```python
from build123d import *

# Parameters (mm, degrees)
SKETCH1_R                = 3
BOSS_EXTRUDE1_DEPTH      = 17
CUT_EXTRUDE3_DEPTH       = 10.2
BOSS_EXTRUDE2_DEPTH      = 2
SKETCH4_R                = 1.5
BOSS_EXTRUDE3_DEPTH      = 18.5
BOSS_EXTRUDE4_DEPTH      = 2
BOSS_EXTRUDE4_DEPTH_BACK = 1
SKETCH6_R                = 2
SKETCH6_R_2              = 1
SKETCH7_R                = 1.1
CUT_EXTRUDE4_DEPTH       = 3


with BuildPart() as part:
    # Sketch1 → Boss-Extrude1 (new body)
    with BuildSketch(Plane(origin=(0, 0, 0), x_dir=(1, 0, 0), z_dir=(0, 1, 0))):
        with Locations(Location((0, 0, 0), (0, 0, 270))):
            Circle(SKETCH1_R)
    extrude(amount=BOSS_EXTRUDE1_DEPTH)

    # Sketch2 → Cut-Extrude3 (cut)
    with BuildSketch(Plane(origin=(0, 17, 0), x_dir=(1, 0, 0), z_dir=(0, 1, 0))):
        with BuildLine():
            Line((1.2, 1.204159458), (1.2, -1.204159458))
            ThreePointArc((1.2, -1.204159458), (-1.7, 0), (1.2, 1.204159458))
        make_face()
    extrude(amount=-CUT_EXTRUDE3_DEPTH, mode=Mode.SUBTRACT)

    # Sketch3 → Boss-Extrude2 (add)
    with BuildSketch(Plane(origin=(0, 0, 0), x_dir=(-1, 0, 0), z_dir=(0, -1, 0))):
        Polygon((5.196152423, 0), (2.598076211, 4.5), (-2.598076211, 4.5), (-5.196152423, 0), (-2.598076211, -4.5), (2.598076211, -4.5), align=None)
    extrude(amount=-BOSS_EXTRUDE2_DEPTH)

    # Sketch4 → Boss-Extrude3 (add)
    with BuildSketch(Plane(origin=(0, 0, 0), x_dir=(-1, 0, 0), z_dir=(0, -1, 0))):
        with Locations(Location((0, 0, 0), (0, 0, 90))):
            Circle(SKETCH4_R)
    extrude(amount=BOSS_EXTRUDE3_DEPTH)

    # Sketch6 → Boss-Extrude4 (add, two sides: drawn at the far end of the back side and taken through both)
    with BuildSketch(Plane(origin=(3, 0, 0), x_dir=(0, 0, -1), z_dir=(1, 0, 0)).offset(-BOSS_EXTRUDE4_DEPTH_BACK)):
        with Locations((0, 12)):
            Circle(SKETCH6_R)
        with Locations((0, 12)):
            Circle(SKETCH6_R_2, mode=Mode.SUBTRACT)
    extrude(amount=BOSS_EXTRUDE4_DEPTH + BOSS_EXTRUDE4_DEPTH_BACK)

    # Sketch7 → Cut-Extrude4 (cut)
    with BuildSketch(Plane(origin=(3, 0, 0), x_dir=(0, 0, -1), z_dir=(1, 0, 0))):
        with Locations((0, 12)):
            Circle(SKETCH7_R)
    extrude(amount=-CUT_EXTRUDE4_DEPTH, mode=Mode.SUBTRACT)


solid = part.part
```
For this review, take the finished solid that the model builds, in its own axes (mm). A direction names the side the tool comes from. Give positions to 0.01 mm unless a question says otherwise; leave off trailing zeros. Write each loop counter-clockwise with the first axis right and the second up, starting at its lowest first coordinate (ties: lowest second). Pieces come first, ordered by that corner, then holes.
Item 1: Machinability: for faces 5 (the face through (3.906, 10.226, -0.923)), 6 (the face through (-2.93, 9.4, -0.65)), 7 (the face through (-1.7, 11.97, 0.06)), which of the approach directions +Z, -Z, +X, -X, +Y, -Y give a long, thin tool a straight path to every point of the face, cutting with its end or side? Answer none if there is none.
Item 2: Wall thickness on probe 1 along Z at (x, y) = (0, 11.5); probe 2 along X at (y, z) = (13.5, 0); probe 3 along Z at (x, y) = (3.95, 12): over which ranges is each line inside the solid? List them lowest first.
Item 3: Take a section at A-A (y = 12). Give the boundary of the cut face in (x, z), and give its area (3 significant figures).
Item 4: Insertion check: P1, Ø2.5, axis at y = 12, z = 0, coming from the -X side; P2, Ø3, axis at y = 12.5, z = -0.5, coming from the +X side; P3, Ø1, axis at y = 10, z = -3, coming from the +X side. Each pin has a flat end and moves straight along its axis. Give the tip position at first contact, or say it passes through.
Item 5: Take a section at B-B (x = 0). Give the boundary of the cut face in (y, z).
Item 6: The part is to be moulded in two halves that separate along X. For faces 1 (the face through (2.113, 10.926, 0.238)), 2 (the face through (0, 1, 4.5)), 3 (the face through (-3.915, 0.986, -2.219)), 4 (the face through (0, 6.8, 0)), say which applies: +X half, -X half, draft (parallel to the pull), parting line (faces both ways), or undercut.
Item 7: Take a section at C-C (z = -3.75). Give the boundary of the cut face in (x, y).
Item 8: Take a section at D-D (y = -15). Give the boundary of the cut face in (x, z), and give its area (3 significant figures).
Established:
1. face 5: +X
1. face 6: none
1. face 7: +Y
2. probe 1: z = -3 to -1.7, 1.7 to 3
2. probe 2: x = -3 to -1.7, 1.2 to 5
2. probe 3: z = -2 to -1, 1 to 2
3. outline: (1.2, -1.2) arc R1.7 cw (long way) to (1.2, 1.2) - (1.2, 1.1) - (3, 1.1) - (3, 1) - (5, 1) - (5, 2) - (2.24, 2) arc R3 ccw (long way) to (2.24, -2) - (5, -2) - (5, -1) - (3, -1) - (3, -1.1) - (1.2, -1.1) - close
3. area: 21.0 mm2
4. P1: stops at x = -3
4. P2: stops at x = 5
4. P3: stops at x = 1.66
5. outline: (-18.5, -1.5) - (0, -1.5) - (0, -4.5) - (2, -4.5) - (2, -3) - (17, -3) - (17, -1.7) - (6.8, -1.7) - (6.8, 1.7) - (17, 1.7) - (17, 3) - (2, 3) - (2, 4.5) - (0, 4.5) - (0, 1.5) - (-18.5, 1.5) - close
6. face 1: undercut
6. face 2: draft
6. face 3: -X half
6. face 4: undercut
7. outline: (-3.03, 0) - (3.03, 0) - (3.03, 2) - (-3.03, 2) - close
8. outline: circle Ø3 at (0, 0)
8. area: 7.07 mm2
